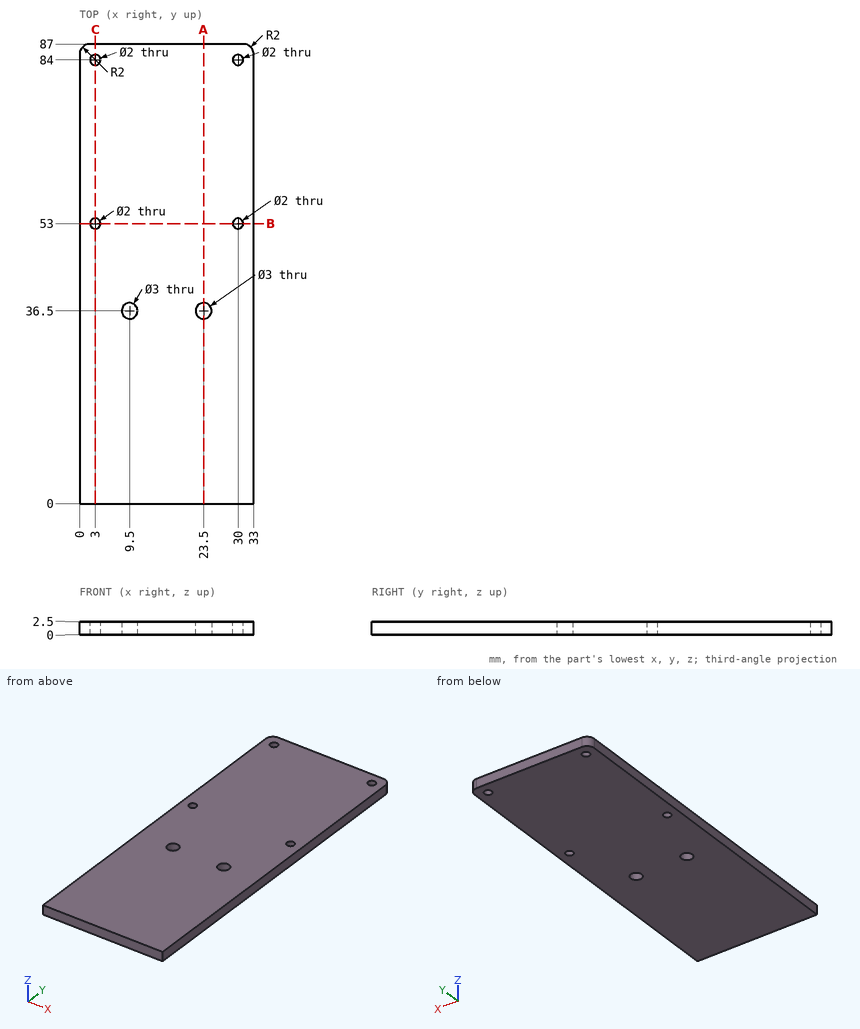
The drawing under review shows one solid part. Ordinate dimensions are in mm from its lowest x, y, z. Coordinates: 2 decimals unless noted, no trailing zeros. Write each loop counter-clockwise with the first axis right and the second up, starting at its lowest first coordinate (ties: lowest second). Pieces come first, ordered by that corner, then holes.
1) Add section B-B (y = 53). Write out the cut boundary in (x, z), plus the area to 3 significant figures.
2) Add section A-A (x = 23.5). Write out the cut boundary in (y, z), plus the area to 3 significant figures.
3) Add section C-C (x = 3). Write out the cut boundary in (y, z), plus the area to 4 significant figures.
4) To check wall thickness, follow L1, parallel to Y at x = 30, z = 0.8; L2, parallel to Y at x = 23.5, z = 0.5; L3, parallel to Y at x = 9, z = 2.4. State the ranges of each line that lie inside material, in increasing order.
5) Insertion check: pin 1 (4 mm diameter, centred on x = 9.5, y = 36.5, fed in from +Z); pin 2 (1.2 mm diameter, centred on x = 3, y = 84, fed in from -Z). Each pin has a flat end and moves straight along its axis. Give the tip position at first contact, or say it passes through.
Check result:
1. outline: (0, 0) - (2, 0) - (2, 2.5) - (0, 2.5) - close; (4, 0) - (29, 0) - (29, 2.5) - (4, 2.5) - close; (31, 0) - (33, 0) - (33, 2.5) - (31, 2.5) - close
1. area: 72.5 mm2
2. outline: (0, 0) - (35, 0) - (35, 2.5) - (0, 2.5) - close; (38, 0) - (87, 0) - (87, 2.5) - (38, 2.5) - close
2. area: 210 mm2
3. outline: (0, 0) - (52, 0) - (52, 2.5) - (0, 2.5) - close; (54, 0) - (83, 0) - (83, 2.5) - (54, 2.5) - close; (85, 0) - (87, 0) - (87, 2.5) - (85, 2.5) - close
3. area: 207.5 mm2
4. L1: y = 0 to 52, 54 to 83, 85 to 87
4. L2: y = 0 to 35, 38 to 87
4. L3: y = 0 to 35.09, 37.91 to 87
5. pin 1: stops at z = 2.5
5. pin 2: passes through
